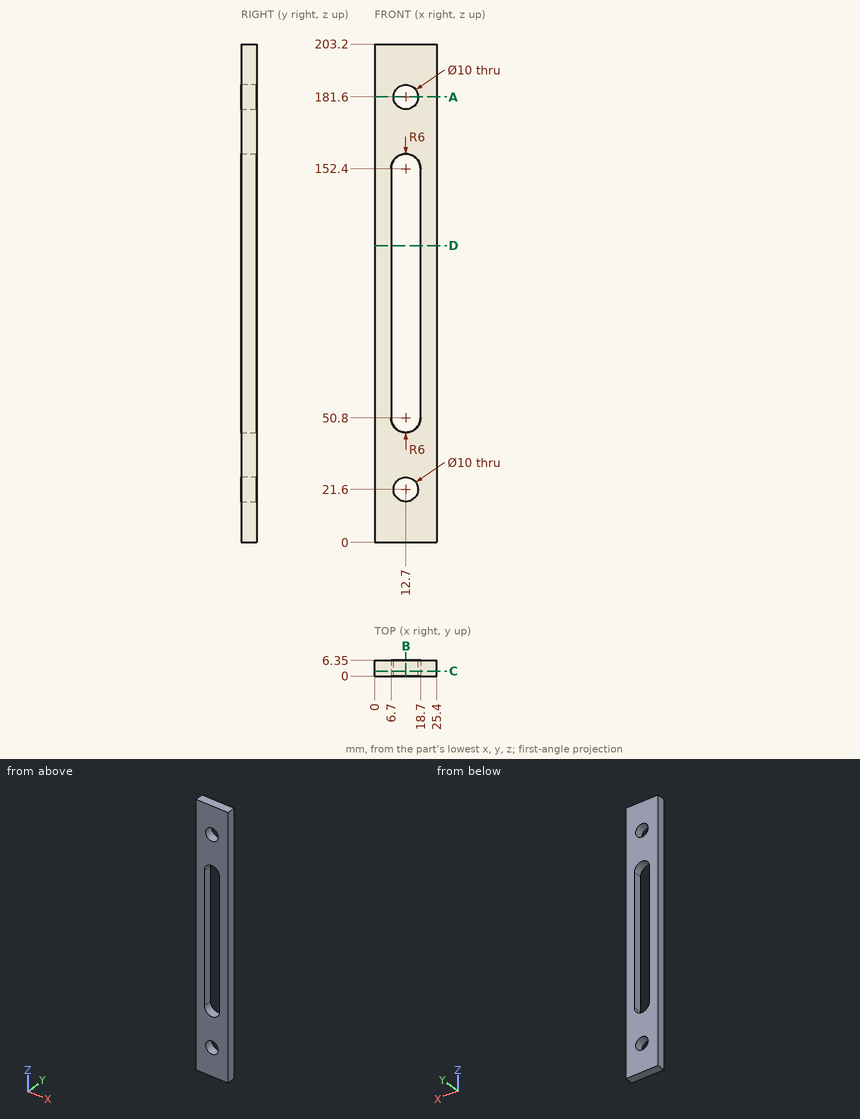
Can you work these out from the drawing? Everything is in mm from the part's minimum corner. Coordinates: 2 decimals unless noted, no trailing zeros. Write each loop counter-clockwise with the first axis right and the second up, starting at its lowest first coordinate (ties: lowest second). Pieces come first, ordered by that corner, then holes. Notation, with made-up numbers: (14, -30) -> (44, -30) arc R24 cw to (44, -16) -> close; hole circle Ø4 at (-24.5, 24.5). An arc over 180 degrees is marked (long way). Write item = value, one per line.
(1) Imagine slicing it at D-D (z = 121). Please give me the cut outline in (x, y), and give its area (3 significant figures).
Verdict:
outline = (0, 0) -> (6.7, 0) -> (6.7, 6.35) -> (0, 6.35) -> close; (18.7, 0) -> (25.4, 0) -> (25.4, 6.35) -> (18.7, 6.35) -> close
area = 85.1 mm^2
(2) Imagine slicing it at A-A (z = 181.6). Please give me the cut outline in (x, y), and give its area (3 significant figures).
Verdict:
outline = (0, 0) -> (7.7, 0) -> (7.7, 6.35) -> (0, 6.35) -> close; (17.7, 0) -> (25.4, 0) -> (25.4, 6.35) -> (17.7, 6.35) -> close
area = 97.8 mm^2
(3) If I drill on probe 1 along X at (y, z) = (0.75, 80); probe 2 along Z at (x, y) = (13.5, 5.5); probe 3 along X at (y, z) = (5.25, 181.6), over which ranges is the centre line in solid material (lowest first)?
Verdict:
probe_1 = 0 to 6.7, 18.7 to 25.4
probe_2 = 0 to 16.66, 26.54 to 44.85, 158.35 to 176.66, 186.54 to 203.2
probe_3 = 0 to 7.7, 17.7 to 25.4
(4) Imagine slicing it at C-C (y = 2). Please give me the cut outline in (x, z), and give its area (3 significant figures).
Verdict:
outline = (0, 0) -> (25.4, 0) -> (25.4, 203.2) -> (0, 203.2) -> close; hole (6.7, 50.8) arc R6 ccw to (18.7, 50.8) -> (18.7, 152.4) arc R6 ccw to (6.7, 152.4) -> close; hole circle Ø10 at (12.7, 21.6); hole circle Ø10 at (12.7, 181.6)
area = 3,670 mm^2
(5) Imagine slicing it at B-B (x = 12.7). Please give me the cut outline in (y, z).
Verdict:
outline = (0, 0) -> (6.35, 0) -> (6.35, 16.6) -> (0, 16.6) -> close; (0, 26.6) -> (6.35, 26.6) -> (6.35, 44.8) -> (0, 44.8) -> close; (0, 158.4) -> (6.35, 158.4) -> (6.35, 176.6) -> (0, 176.6) -> close; (0, 186.6) -> (6.35, 186.6) -> (6.35, 203.2) -> (0, 203.2) -> close
